```python
from build123d import *

# Parameters (mm, degrees)
SKETCH_1_W          = 127.8
SKETCH_1_H          = 7.8
EXTRUDE_1_DEPTH     = 9.6
SKETCH_2_R          = 2.4
EXTRUDE_2_DEPTH     = 1.7
SKETCH_3_R          = 2.5
CUT_EXTRUDE_2_DEPTH = 1.8


with BuildPart() as part:
    # Эскиз1 → Бобышка-Вытянуть1 (new body)
    with BuildSketch(Plane(origin=(0, 0, 0), x_dir=(1, 0, 0), z_dir=(0, 1, 0))):
        Rectangle(SKETCH_1_W, SKETCH_1_H)
    extrude(amount=EXTRUDE_1_DEPTH)

    # Эскиз2 → Бобышка-Вытянуть2 (add)
    with BuildSketch(Plane(origin=(0, 9.6, 0), x_dir=(1, 0, 0), z_dir=(0, 1, 0))):
        with Locations(Location((-60, 0, 0), (0, 0, 90))):
            Circle(SKETCH_2_R)
        with Locations(Location((-52.126, 0, 0), (0, 0, 90))):
            Circle(SKETCH_2_R)
        with Locations(Location((-44.252, 0, 0), (0, 0, 90))):
            Circle(SKETCH_2_R)
        with Locations(Location((-36.378, 0, 0), (0, 0, 90))):
            Circle(SKETCH_2_R)
        with Locations(Location((-28.504, 0, 0), (0, 0, 90))):
            Circle(SKETCH_2_R)
        with Locations(Location((-20.63, 0, 0), (0, 0, 90))):
            Circle(SKETCH_2_R)
        with Locations(Location((-12.756, 0, 0), (0, 0, 90))):
            Circle(SKETCH_2_R)
        with Locations(Location((-4.882, 0, 0), (0, 0, 90))):
            Circle(SKETCH_2_R)
        with Locations(Location((2.992, 0, 0), (0, 0, 90))):
            Circle(SKETCH_2_R)
        with Locations(Location((10.866, 0, 0), (0, 0, 90))):
            Circle(SKETCH_2_R)
        with Locations(Location((18.74, 0, 0), (0, 0, 90))):
            Circle(SKETCH_2_R)
        with Locations(Location((26.614, 0, 0), (0, 0, 90))):
            Circle(SKETCH_2_R)
        with Locations(Location((34.488, 0, 0), (0, 0, 90))):
            Circle(SKETCH_2_R)
        with Locations(Location((42.362, 0, 0), (0, 0, 90))):
            Circle(SKETCH_2_R)
        with Locations(Location((50.236, 0, 0), (0, 0, 90))):
            Circle(SKETCH_2_R)
        with Locations(Location((58.11, 0, 0), (0, 0, 90))):
            Circle(SKETCH_2_R)
    extrude(amount=EXTRUDE_2_DEPTH)

    # Эскиз3 → Вырез-Вытянуть2 (cut)
    with BuildSketch(Plane.XZ):
        with Locations(Location((-60, 0, 0), (0, 0, 270))):
            Circle(SKETCH_3_R)
        with Locations(Location((-52.126, 0, 0), (0, 0, 270))):
            Circle(SKETCH_3_R)
        with Locations(Location((-44.252, 0, 0), (0, 0, 270))):
            Circle(SKETCH_3_R)
        with Locations(Location((-36.378, 0, 0), (0, 0, 270))):
            Circle(SKETCH_3_R)
        with Locations(Location((-28.504, 0, 0), (0, 0, 270))):
            Circle(SKETCH_3_R)
        with Locations(Location((-20.63, 0, 0), (0, 0, 270))):
            Circle(SKETCH_3_R)
        with Locations(Location((-12.756, 0, 0), (0, 0, 270))):
            Circle(SKETCH_3_R)
        with Locations(Location((-4.882, 0, 0), (0, 0, 270))):
            Circle(SKETCH_3_R)
        with Locations(Location((2.992, 0, 0), (0, 0, 270))):
            Circle(SKETCH_3_R)
        with Locations(Location((10.866, 0, 0), (0, 0, 270))):
            Circle(SKETCH_3_R)
        with Locations(Location((18.74, 0, 0), (0, 0, 270))):
            Circle(SKETCH_3_R)
        with Locations(Location((26.614, 0, 0), (0, 0, 270))):
            Circle(SKETCH_3_R)
        with Locations(Location((34.488, 0, 0), (0, 0, 270))):
            Circle(SKETCH_3_R)
        with Locations(Location((42.362, 0, 0), (0, 0, 270))):
            Circle(SKETCH_3_R)
        with Locations(Location((50.236, 0, 0), (0, 0, 270))):
            Circle(SKETCH_3_R)
        with Locations(Location((58.11, 0, 0), (0, 0, 270))):
            Circle(SKETCH_3_R)
    extrude(amount=-CUT_EXTRUDE_2_DEPTH, mode=Mode.SUBTRACT)


solid = part.part
```
Read the model definition and answer for the solid it produces. Units are mm, in the model's axes. A direction names the side the tool comes from. Coordinates: 2 decimals unless noted, no trailing zeros. Loops run counter-clockwise (first coordinate to the right, second up) from the corner with the lowest first, then second, coordinate; pieces in that order, holes last.
(1) The part is cut by section A-A (x = 58.11). Determine the outline of the cut face in (y, z).
Solution:
outline: (0, -3.9) - (9.6, -3.9) - (9.6, -2.4) - (11.3, -2.4) - (11.3, 2.4) - (9.6, 2.4) - (9.6, 3.9) - (0, 3.9) - (0, 2.5) - (1.8, 2.5) - (1.8, -2.5) - (0, -2.5) - close
(2) A flat-ended cylindrical pin translates along its axis: pin 1 Ø1.5 at (x, z) = (10.5, -0.5) entering from -Y. Find the tip coordinate at first contact, or state that the pin passes through.
Solution:
pin 1: stops at y = 1.8
(3) The mould has two halves that part along X. Classify faces 4 (the face through (11, 1.8, 0)), 5 (the face through (-1, 0, 0)): released by +X, released by -X, zero draft, split by the parting line, or undercut.
Solution:
face 4: undercut
face 5: zero draft
(4) Consider line 1 along Y through (x, z) = (-32.5, 3); line 2 along Y through (x, z) = (-45.5, 1); line 3 along Z through (x, y) = (11, 9.75). Determine where each line is inside the solid, lowest interval first.
Solution:
line 1: y = 0 to 9.6
line 2: y = 1.8 to 11.3
line 3: z = -2.4 to 2.4
(5) A tool of negligible diameter and unlimited length cuts with its end or side. For faces 1 (the face through (-10.63, 10.44, -1.11)), 2 (the face through (27, 1.8, 0)), 3 (the face through (-60, 11.3, 0)), from which of +Z, -Z, +X, -X, +Y, -Y can it reach the whole face along a straight path? Write none if from no direction.
Solution:
face 1: +Y
face 2: -Y
face 3: +Z, -Z, +X, -X, +Y
(6) The part is cut by section B-B (x = 12). Determine the outline of the cut face in (y, z), and give its area (3 significant figures).
Solution:
outline: (0, -3.9) - (9.6, -3.9) - (9.6, -2.12) - (11.3, -2.12) - (11.3, 2.12) - (9.6, 2.12) - (9.6, 3.9) - (0, 3.9) - (0, 2.23) - (1.8, 2.23) - (1.8, -2.23) - (0, -2.23) - close
area: 74.1 mm2
